from build123d import *

# Parameters (mm, degrees)
SKETCH1_W           = 95
SKETCH1_H           = 57
SKETCH1_R           = 2.057983022
BOSS_EXTRUDE2_DEPTH = 12
BOSS_EXTRUDE3_DEPTH = 9.5


with BuildPart() as part:
    # Sketch1 → Boss-Extrude2 (new body)
    with BuildSketch(Plane(origin=(0, 0, 0), x_dir=(1, 0, 0), z_dir=(0, 1, 0))):
        Rectangle(SKETCH1_W, SKETCH1_H)
        with Locations(Location((41.5, 22.5, 0), (0, 0, 270))):
            Circle(SKETCH1_R, mode=Mode.SUBTRACT)
        with Locations(Location((-41.5, 22.5, 0), (0, 0, 270))):
            Circle(SKETCH1_R, mode=Mode.SUBTRACT)
        with Locations(Location((41.5, -22.5, 0), (0, 0, 270))):
            Circle(SKETCH1_R, mode=Mode.SUBTRACT)
        with Locations(Location((-41.5, -22.5, 0), (0, 0, 270))):
            Circle(SKETCH1_R, mode=Mode.SUBTRACT)
        with BuildLine():
            Line((-37, 12.5), (-37, -12.5))
            ThreePointArc((-37, -12.5), (-36.853553391, -12.853553391), (-36.5, -13))
            Line((-36.5, -13), (32.5, -13))
            ThreePointArc((32.5, -13), (32.853553391, -12.853553391), (33, -12.5))
            Line((33, -12.5), (33, 12.5))
            ThreePointArc((33, 12.5), (32.853553391, 12.853553391), (32.5, 13))
            Line((32.5, 13), (-36.5, 13))
            ThreePointArc((-36.5, 13), (-36.853553391, 12.853553391), (-37, 12.5))
        make_face(mode=Mode.SUBTRACT)
    extrude(amount=BOSS_EXTRUDE2_DEPTH)

    # Sketch1_5 → Boss-Extrude3 (add)
    with BuildSketch(Plane(origin=(0, 0, 0), x_dir=(1, 0, 0), z_dir=(0, 1, 0))):
        with BuildLine():
            ThreePointArc((-37, 12.5), (-36.853553391, 12.853553391), (-36.5, 13))
            Line((-36.5, 13), (32.5, 13))
            ThreePointArc((32.5, 13), (32.853553391, 12.853553391), (33, 12.5))
            Line((33, 12.5), (33, -12.5))
            ThreePointArc((33, -12.5), (32.853553391, -12.853553391), (32.5, -13))
            Line((32.5, -13), (-36.5, -13))
            ThreePointArc((-36.5, -13), (-36.853553391, -12.853553391), (-37, -12.5))
            Line((-37, -12.5), (-37, 12.5))
        make_face()
        with BuildLine():
            ThreePointArc((30, -10), (30.353553391, -9.853553391), (30.5, -9.5))
            Line((30.5, -9.5), (30.5, 9.5))
            ThreePointArc((30.5, 9.5), (30.353553391, 9.853553391), (30, 10))
            Line((30, 10), (-34, 10))
            ThreePointArc((-34, 10), (-34.353553391, 9.853553391), (-34.5, 9.5))
            Line((-34.5, 9.5), (-34.5, -9.5))
            ThreePointArc((-34.5, -9.5), (-34.353553391, -9.853553391), (-34, -10))
            Line((-34, -10), (30, -10))
        make_face(mode=Mode.SUBTRACT)
    extrude(amount=BOSS_EXTRUDE3_DEPTH)


solid = part.part
Source: CAD feature listing. Evaluate the final solid. Frame: model axes, mm. A direction names the side the tool comes from. Give positions to 0.01 mm unless a question says otherwise; leave off trailing zeros. Order: outer loops, then holes, each group sorted by start corner. A loop starts at its lowest first (then second) coordinate and runs counter-clockwise, first axis right, second up. Notation, with made-up numbers: (26.5, -13.5) -> (83.5, -13.5) arc R34 ccw to (83.5, 22.5) -> close; hole circle Ø7 at (85, -32). An arc over 180 degrees is marked (long way). Write item = value, one per line.
Q1. Cut plane D-D, the plane x = 41.5. Output: boundary loops of the cut face in (y, z), and give its area (3 significant figures).
Data:
outline = (0, -28.5) -> (12, -28.5) -> (12, -24.56) -> (0, -24.56) -> close; (0, -20.44) -> (12, -20.44) -> (12, 20.44) -> (0, 20.44) -> close; (0, 24.56) -> (12, 24.56) -> (12, 28.5) -> (0, 28.5) -> close
area = 585 mm^2
Q2. Material intervals for line 1 (X direction, y = 7, z = 22.5); line 2 (X direction, y = 4.5, z = 7); line 3 (Z direction, x = 40.5, y = 5.5), sorted ascending. Write a range as from..to.
Data:
line_1 = -47.5..-43.56, -39.44..39.44, 43.56..47.5
line_2 = -47.5..-34.5, 30.5..47.5
line_3 = -28.5..-24.3, -20.7..20.7, 24.3..28.5
Q3. Cut plane A-A, the plane x = 4.5. Output: boundary loops of the cut face in (y, z).
Data:
outline = (0, -28.5) -> (12, -28.5) -> (12, -13) -> (9.5, -13) -> (9.5, -10) -> (0, -10) -> close; (0, 10) -> (9.5, 10) -> (9.5, 13) -> (12, 13) -> (12, 28.5) -> (0, 28.5) -> close
Q4. Pin query (flat end, axial travel): pin 1 (8 mm diameter, centred on x = -6, z = 4.5, fed in from +Y); pin 2 (4.5 mm diameter, centred on x = 41.5, z = 22.5, fed in from +Y). Return the tip coordinate at first contact, or that it passes through.
Data:
pin_1 = through
pin_2 = 12
Q5. Cut plane C-C, the plane z = -22.5. Output: boundary loops of the cut face in (x, y), and give its area (3 significant figures).
Data:
outline = (-47.5, 0) -> (-43.56, 0) -> (-43.56, 12) -> (-47.5, 12) -> close; (-39.44, 0) -> (39.44, 0) -> (39.44, 12) -> (-39.44, 12) -> close; (43.56, 0) -> (47.5, 0) -> (47.5, 12) -> (43.56, 12) -> close
area = 1,040 mm^2
Q6. Cut plane B-B, the plane y = 11. Output: boundary loops of the cut face in (x, z).
Data:
outline = (-47.5, -28.5) -> (47.5, -28.5) -> (47.5, 28.5) -> (-47.5, 28.5) -> close; hole circle Ø4.12 at (-41.5, -22.5); hole circle Ø4.12 at (-41.5, 22.5); hole (-37, -12.5) arc R0.5 ccw to (-36.5, -13) -> (32.5, -13) arc R0.5 ccw to (33, -12.5) -> (33, 12.5) arc R0.5 ccw to (32.5, 13) -> (-36.5, 13) arc R0.5 ccw to (-37, 12.5) -> close; hole circle Ø4.12 at (41.5, -22.5); hole circle Ø4.12 at (41.5, 22.5)
Q7. Pull-direction query (Z, two-part tool) for faces 1 (the face through (-2, 5, 10)), 2 (the face through (-1, 6, 28.5)), 3 (the face through (47.5, 6, 0)); classes: released by +Z, released by -Z, zero draft, split by the parting line, or undercut.
Data:
face_1 = undercut
face_2 = released by +Z
face_3 = zero draft
Q8. Set-up query: faces 4 (the face through (-47.5, 6, 0)), 5 (the face through (-34.5, 5, 0)), 6 (the face through (-2, 11, 13)). Return all of +Z, -Z, +X, -X, +Y, -Y with unobstructed straight access to the full face (end or side cutting, diameter ignored); none if empty.
Data:
face_4 = +Z, -Z, -X, +Y, -Y
face_5 = +Y, -Y
face_6 = +Y
